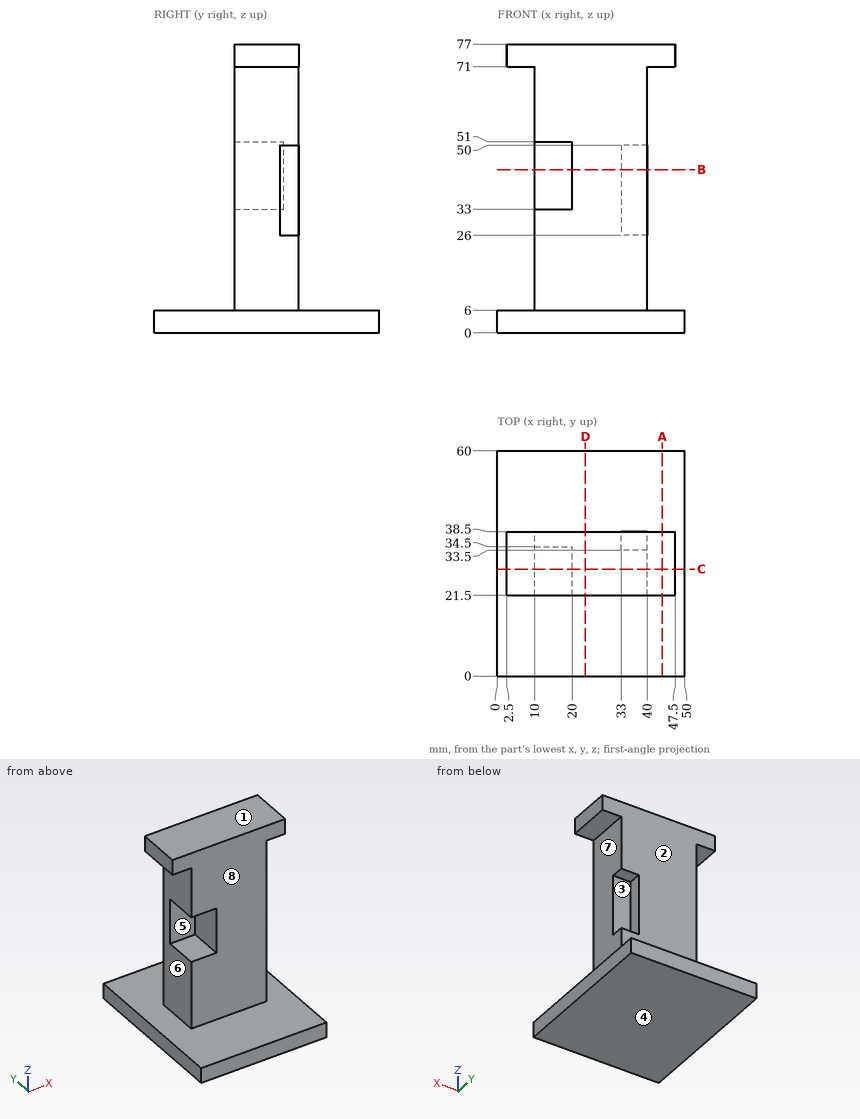
For this review, use the dimensioned drawing (mm, ordinates from the lowest corner) and the shaded views. A direction names the side the tool comes from. Give positions to 0.01 mm unless a question says otherwise; leave off trailing zeros. Order: outer loops, then holes, each group sorted by start corner. A loop starts at its lowest first (then second) coordinate and runs counter-clockwise, first axis right, second up. Notation, with made-up numbers: M 67,74 L 107,74 A16 ccw 107,84 Z; hole C 30,21.5 d3. An arc over 180 degrees is marked long. Use one line per item in the form item = value. Start each with the question number.
Item 1: Insertion check: pin 1 Ø1 at (y, z) = (32, 67) entering from +X; pin 2 Ø1.5 at (x, z) = (17.5, 30) entering from +Y; pin 3 Ø6 at (x, y) = (7.5, 49) entering from +Z. Each pin has a flat end and moves straight along its axis. Give the tip position at first contact, or say it passes through.
Item 2: For the marked faces 4, 5, 6, 7 and 8, list the 3-axis set-ups (+Z, -Z, +X, -X, +Y, -Y) from which the entire face can be reached by the end or side of a thin tool; tool diameter is ignored.
Item 3: The part is to be moulded in two halves that separate along Z. For the marked faces 1, 2 and 3, say which applies: pulls with the +Z half, pulls with the -Z half, needs draft (parallel to the pull), parting line crosses it, or undercut.
Item 4: We need section A-A on x = 44. Give the boundary of the cut face in (y, z), plus the area to 3 significant figures.
Item 5: We need section D-D on x = 23.5. Give the boundary of the cut face in (y, z).
Item 6: We need section C-C on y = 28.5. Give the boundary of the cut face in (x, z).
Item 7: To check wall thickness, follow line 1 along Z through (x, y) = (37, 38); line 2 along Y through (x, z) = (20.5, 33.5); line 3 along Z through (x, y) = (20, 43). State the ranges of each line that lie inside material, in increasing order. Write a range as from..to.
Item 8: We need section B-B on z = 43.5. Give the boundary of the cut face in (x, y).
Completed:
q1.pin_1 = 40
q1.pin_2 = 38.5
q1.pin_3 = 6
q2.face_4 = -Z, +X, -X, +Y, -Y
q2.face_5 = -X, -Y
q2.face_6 = -X, +Y, -Y
q2.face_7 = +X, +Y, -Y
q2.face_8 = +Z, +X, -X, -Y
q3.face_1 = pulls with the +Z half
q3.face_2 = needs draft
q3.face_3 = undercut
q4.outline = M 0,0 L 60,0 L 60,6 L 0,6 Z; M 21.5,71 L 38.5,71 L 38.5,77 L 21.5,77 Z
q4.area = 462 mm²
q5.outline = M 0,0 L 60,0 L 60,6 L 38.5,6 L 38.5,77 L 21.5,77 L 21.5,6 L 0,6 Z
q6.outline = M 0,0 L 50,0 L 50,6 L 40,6 L 40,71 L 47.5,71 L 47.5,77 L 2.5,77 L 2.5,71 L 10,71 L 10,51 L 20,51 L 20,33 L 10,33 L 10,6 L 0,6 Z
q7.line_1 = 0..26, 50..77
q7.line_2 = 21.5..38.5
q7.line_3 = 0..6
q8.outline = M 10,34.5 L 20,34.5 L 20,21.5 L 40,21.5 L 40,33.5 L 33,33.5 L 33,38.5 L 10,38.5 Z
